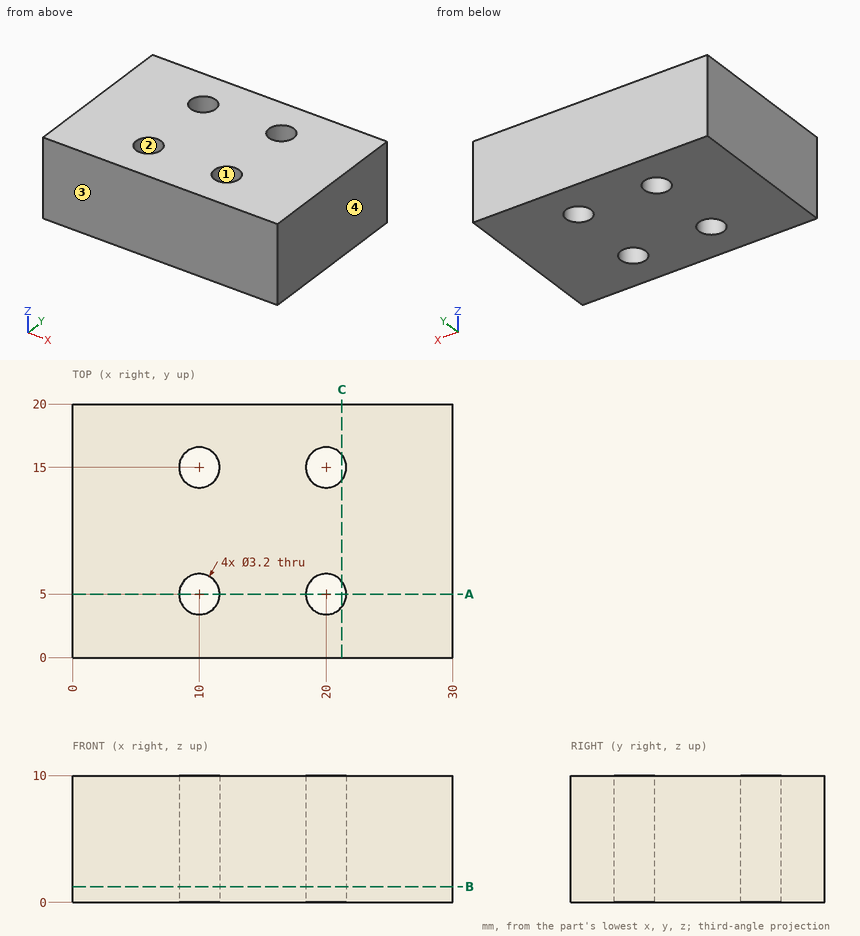
Check sheet for the drawn part. Datum: minimum x, y, z corner. Units: mm. Coordinates: 2 decimals unless noted, no trailing zeros. Order: outer loops, then holes, each group sorted by start corner. A loop starts at its lowest first (then second) coordinate and runs counter-clockwise, first axis right, second up. Notation, with made-up numbers: (-34, 55) -> (-30, 55) arc R25 ccw to (-30, 77) -> close; hole circle Ø9 at (75.25, -7.5). An arc over 180 degrees is marked (long way). Use a Markdown table: item, result. Add a question column.
1. Cross-section at C-C (x = 21.25). Enter the section's corners in (y, z).
2. Cross-section at B-B (z = 1.25). Enter the section's corners in (x, y), and give its area (3 significant figures).
3. Cross-section at A-A (y = 5). Enter the section's corners in (x, z), and give its area (3 significant figures).
4. Material ranges on L1, parallel to Y at x = 20, z = 5.75; L2, parallel to Y at x = 9, z = 6.5; L3, parallel to X at y = 14.5, z = 5.25, recorded low to high.
5. Mould release check, pull along X, two halves, no side actions. Record for the marked faces 1, 2, 3 and 4: pulls with the +X half, pulls with the -X half, needs draft (parallel to the pull), parting line crosses it, or undercut.
Filled sheet:
| question | item | result |
|---|---|---|
| 1 | outline | (0, 0) -> (4, 0) -> (4, 10) -> (0, 10) -> close; (6, 0) -> (14, 0) -> (14, 10) -> (6, 10) -> close; (16, 0) -> (20, 0) -> (20, 10) -> (16, 10) -> close |
| 2 | outline | (0, 0) -> (30, 0) -> (30, 20) -> (0, 20) -> close; hole circle Ø3.2 at (10, 5); hole circle Ø3.2 at (10, 15); hole circle Ø3.2 at (20, 5); hole circle Ø3.2 at (20, 15) |
| 2 | area | 568 mm2 |
| 3 | outline | (0, 0) -> (8.4, 0) -> (8.4, 10) -> (0, 10) -> close; (11.6, 0) -> (18.4, 0) -> (18.4, 10) -> (11.6, 10) -> close; (21.6, 0) -> (30, 0) -> (30, 10) -> (21.6, 10) -> close |
| 3 | area | 236 mm2 |
| 4 | L1 | 0 to 3.4, 6.6 to 13.4, 16.6 to 20 |
| 4 | L2 | 0 to 3.75, 6.25 to 13.75, 16.25 to 20 |
| 4 | L3 | 0 to 8.48, 11.52 to 18.48, 21.52 to 30 |
| 5 | face 1 | undercut |
| 5 | face 2 | undercut |
| 5 | face 3 | needs draft |
| 5 | face 4 | pulls with the +X half |
